Input: dimensioned drawing with shaded views. Units: mm. Origin: part minimum x, y, z. Give positions to 0.01 mm unless a question says otherwise; leave off trailing zeros. Loops run counter-clockwise (first coordinate to the right, second up) from the corner with the lowest first, then second, coordinate; pieces in that order, holes last. Notation, with made-up numbers: M -18,30 L 2,30 A37 ccw 2,67 Z; hole C -20.75,60.5 d5. An arc over 180 degrees is marked long. Use CSV: the item, a comma, the result in double quotes. Start each with the question number.
Q1. Section B-B, the plane z = 5. Output: boundary loops of the cut face in (x, y).
Q2. Section A-A, the plane x = 5. Output: boundary loops of the cut face in (y, z), plus the area to 3 significant figures.
Q3. Material intervals for line 1 along Z through (x, y) = (115, 0.4); line 2 along Z through (x, y) = (115, 3.05), sorted ascending.
Q4. Pin query (flat end, axial travel): pin 1 (1.8 mm diameter, centred on x = 6.5, z = 34.5, fed in from -Y). Return the tip coordinate at first contact, or that it passes through.
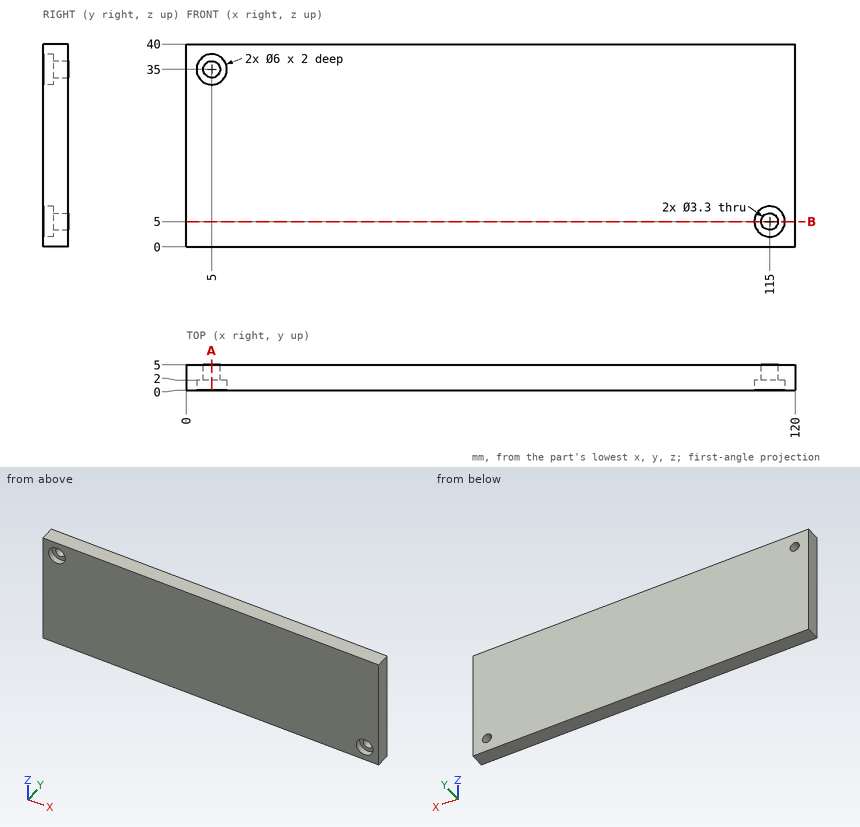
A:
1,outline,"M 0,0 L 112,0 L 112,2 L 113.35,2 L 113.35,5 L 0,5 Z; M 116.65,2 L 118,2 L 118,0 L 120,0 L 120,5 L 116.65,5 Z"
2,outline,"M 0,0 L 5,0 L 5,33.35 L 2,33.35 L 2,32 L 0,32 Z; M 0,38 L 2,38 L 2,36.65 L 5,36.65 L 5,40 L 0,40 Z"
2,area,"178 mm^2"
3,line 1,"0 to 2, 8 to 40"
3,line 2,"0 to 3.35, 6.65 to 40"
4,pin 1,"y = 2"
